Source: CAD feature listing. Evaluate the final solid. Frame: model axes, mm. A direction names the side the tool comes from. Give positions to 0.01 mm unless a question says otherwise; leave off trailing zeros. Write each loop counter-clockwise with the first axis right and the second up, starting at its lowest first coordinate (ties: lowest second). Pieces come first, ordered by that corner, then holes. Notation, with made-up numbers: (-2, 29.5) -> (16, 29.5) arc R10 ccw to (16, 40.5) -> close; hole circle Ø2 at (-9.5, -32). An arc over 180 degrees is marked (long way). Use one line per item in the form item = value. Start each with the question number.
(1) Cut plane C-C, the plane x = 62. Output: boundary loops of the cut face in (y, z), and give its area (3 significant figures).
(2) Cut plane B-B, the plane y = 17. Output: boundary loops of the cut face in (x, z), and give its area (3 significant figures).
(3) Set-up query: faces 1 (the face through (64.5, -49, 157)), 2 (the face through (-1, 60.5, 149)), 3 (the face through (-79, -46, 161.5)). Return all of +Z, -Z, +X, -X, +Y, -Y with unobstructed straight access to the full face (end or side cutting, diameter ignored); none if empty.
(4) Material intervals for line 1 along Z through (x, y) = (-2, 47.5); line 2 along Z through (x, y) = (79, -46.5); line 3 along X through (y, z) = (24, 148), sorted ascending. Write a range as from..to.
(5) Draft query along X for faces 4 (the face through (1, -60.5, 150)), 5 (the face through (-93.5, -14, 150)), 6 (the face through (-79.319, -22.504, 157.19)). Return one class per face: pulls with the +X half, pulls with the -X half, needs draft (parallel to the pull), parting line crosses it, or undercut.
(6) Cut plane A-A, the plane x = -79. Output: boundary loops of the cut face in (y, z).
(7) First-contact query: P1, Ø3.5, axis at x = -44.5, z = 148.5, coming from the +Y side; P2, Ø9.5, axis at y = -54, z = 157, coming from the +X side; P3, Ø17.5, axis at y = -11, z = 155, coming from the -X side. Flat tips, straight axial feed; report the tip coordinate or a pass-through.
(8) Cut plane D-D, the plane y = -33. Output: boundary loops of the cut face in (x, z).
Autodesk Fusion 360 part; units mm, degrees
sketch "Sketch1" plane through (0, 0, 0) normal (0, 0, 1) x (1, 0, 0)
  line L0 (96, -63) -> (-96, -63)
  line L1 (-96, -63) -> (-96, 63)
  line L2 (-96, 63) -> (96, 63)
  line L3 (96, 63) -> (96, -63)
  line L4 (96, -63) -> (-96, 63) construction
  line L5 (-96, -63) -> (96, 63) construction
  dimension "d1" = 192
  dimension "d2" = 126
extrude "Extrude1" add sketch "Sketch1" along normal blind 145.75
sketch "Sketch4" plane through (0, 0, 145.75) normal (0, 0, 1) x (-1, 0, 0)
  line L0 (-96, -63) -> (96, -63)
  line L1 (96, -63) -> (96, 63)
  line L2 (96, 63) -> (-96, 63)
  line L3 (-96, 63) -> (-96, -63)
  line L4 (96, -63) -> (-96, -63)
  line L5 (-96, -63) -> (-96, 63)
  line L6 (-96, 63) -> (96, 63)
  line L7 (96, 63) -> (96, -63)
  line L8 (-93.5, 60.5) -> (93.5, 60.5)
  line L9 (93.5, 60.5) -> (93.5, -60.5)
  line L10 (93.5, -60.5) -> (-93.5, -60.5)
  line L11 (-93.5, -60.5) -> (-93.5, 60.5)
  dimension "d12" = 2.5
extrude "Extrude4" add sketch "Sketch4" along normal blind 7.25 contours L8 L9 L10 L11
sketch "Sketch5" plane through (0, 0, 153) normal (0, 0, 1) x (-1, 0, 0)
  line L0 (-93.5, -60.5) -> (93.5, -60.5)
  line L1 (93.5, -60.5) -> (93.5, 60.5)
  line L2 (93.5, 60.5) -> (-93.5, 60.5)
  line L3 (-93.5, 60.5) -> (-93.5, -60.5)
  line L4 (93.5, 60.5) -> (64.5, 60.5)
  line L5 (64.5, 60.5) -> (64.5, 37)
  line L6 (93.5, 37) -> (93.5, 60.5)
  line L7 (-93.5, 60.5) -> (-64.5, 60.5)
  line L8 (-64.5, 60.5) -> (-64.5, 37)
  line L9 (-93.5, 37) -> (-93.5, 60.5)
  arc A0 (64.5, 37) -> (93.5, 37) centre (79, 37) ccw
  arc A1 (-93.5, 37) -> (-64.5, 37) centre (-79, 37) ccw
  dimension "d15" = 14.5
  dimension "d16" = 23.5
extrude "Extrude5" add sketch "Sketch5" along normal blind 8.5 contours L2 L3 L7 L8 L9 A1 | L1 L2 L4 L5 L6 A0
sketch "Sketch6" plane through (0, 0, 161.5) normal (0, 0, 1) x (-1, 0, 0)
  arc A0 (64.5, 37) -> (93.5, 37) centre (79, 37) ccw
  line L0 (93.5, 37) -> (93.5, 60.5)
  line L1 (93.5, 60.5) -> (64.5, 60.5)
  line L2 (64.5, 60.5) -> (64.5, 37)
  circle A1 centre (79, 37) radius 8
  circle A2 centre (-79, 37) radius 8
  arc A3 (-93.5, 37) -> (-64.5, 37) centre (-79, 37) ccw
  dimension "d19" = 16
extrude "Extrude6" add sketch "Sketch6" along normal blind 4.6 contours A1 | A2
equation "d3 = 153 mm - 7.25 mm"
equation "d16 = 38 mm - 14.5 mm"
Geometry says:
q1.outline = (-63, 0) -> (63, 0) -> (63, 145.75) -> (60.5, 145.75) -> (60.5, 153) -> (-60.5, 153) -> (-60.5, 145.75) -> (-63, 145.75) -> close
q1.area = 19,200 mm^2
q2.outline = (-96, 0) -> (96, 0) -> (96, 145.75) -> (93.5, 145.75) -> (93.5, 153) -> (-93.5, 153) -> (-93.5, 145.75) -> (-96, 145.75) -> close
q2.area = 29,300 mm^2
q3.face_1 = +Z, +Y, -Y
q3.face_2 = +Z, +X, -X, +Y
q3.face_3 = +Z
q4.line_1 = 0..153
q4.line_2 = 0..161.5
q4.line_3 = -93.5..93.5
q5.face_4 = needs draft
q5.face_5 = pulls with the -X half
q5.face_6 = undercut
q6.outline = (-63, 0) -> (63, 0) -> (63, 145.75) -> (60.5, 145.75) -> (60.5, 153) -> (-22.5, 153) -> (-22.5, 161.5) -> (-29, 161.5) -> (-29, 166.1) -> (-45, 166.1) -> (-45, 161.5) -> (-60.5, 161.5) -> (-60.5, 145.75) -> (-63, 145.75) -> close
q7.P1 = 60.5
q7.P2 = 93.5
q7.P3 = -93.5
q8.outline = (-96, 0) -> (96, 0) -> (96, 145.75) -> (93.5, 145.75) -> (93.5, 153) -> (92.94, 153) -> (92.94, 161.5) -> (85.93, 161.5) -> (85.93, 166.1) -> (72.07, 166.1) -> (72.07, 161.5) -> (65.06, 161.5) -> (65.06, 153) -> (-65.06, 153) -> (-65.06, 161.5) -> (-72.07, 161.5) -> (-72.07, 166.1) -> (-85.93, 166.1) -> (-85.93, 161.5) -> (-92.94, 161.5) -> (-92.94, 153) -> (-93.5, 153) -> (-93.5, 145.75) -> (-96, 145.75) -> close
